from build123d import *

# Parameters (mm, degrees)
SKETCH1_R           = 12.5
BOSS_EXTRUDE1_DEPTH = 22.6
SKETCH2_R           = 13.5
BOSS_EXTRUDE2_DEPTH = 11.58
SKETCH9_W           = 1.365
SKETCH9_H           = 0.55
SKETCH4_R           = 2.575
MAGNETSLOT_DEPTH    = 1
NUTCUT_DEPTH        = 30.18
SKETCH7_R           = 3.5
NUTHOLE_DEPTH       = 15
SKETCH8_R           = 1.35
SCREWHOLE_DEPTH     = 40.150637287
CIRPATTERN1_COUNT   = 4
SKETCH11_W          = 15.473481632
SKETCH11_H          = 6.154945972
CUT_EXTRUDE1_DEPTH  = 34.488804099


with BuildPart() as part:
    # Sketch1 → Boss-Extrude1 (new body)
    with BuildSketch(Plane.XY):
        Circle(SKETCH1_R)
    extrude(amount=BOSS_EXTRUDE1_DEPTH)

    # Sketch2 → Boss-Extrude2 (add)
    with BuildSketch(Plane.XY):
        Circle(SKETCH2_R)
    extrude(amount=-BOSS_EXTRUDE2_DEPTH)

    # Sketch9 → Cut-Revolve1 (revolve, cut)
    with BuildSketch(Plane(origin=(0, 0, 0), x_dir=(0, 0, -1), z_dir=(1, 0, 0)), mode=Mode.PRIVATE) as cut_revolve1_sk:
        with Locations((-20.6825, -12.225)):
            Rectangle(SKETCH9_W, SKETCH9_H)
    revolve(cut_revolve1_sk.sketch.rotate(Axis((0, 0, 24.309), (0, 0, -1)), 270), axis=Axis((0, 0, 24.309), (0, 0, -1)), mode=Mode.SUBTRACT)

    # Sketch4 → MagnetSlot (cut)
    with BuildSketch(Plane.XY.offset(22.6)):
        Circle(SKETCH4_R)
    magnetslot = extrude(amount=-MAGNETSLOT_DEPTH, mode=Mode.SUBTRACT)

    # Sketch6 → NutCut (cut)
    with BuildSketch(Plane.XY.offset(22.6)):
        Polygon((6.206811366, 8.288877648), (3.362655934, 7.526788497), (2.600566782, 4.682633064), (4.682633064, 2.600566782), (7.526788497, 3.362655934), (8.288877648, 6.206811366), align=None)
    nutcut = extrude(amount=-NUTCUT_DEPTH, mode=Mode.SUBTRACT)

    # Sketch7 → NutHole (cut)
    with BuildSketch(Plane.XY.offset(22.6)):
        with Locations((5.444722215, 5.444722215)):
            Circle(SKETCH7_R)
    nuthole = extrude(amount=-NUTHOLE_DEPTH, mode=Mode.SUBTRACT)

    # Sketch8 → ScrewHole (cut, symmetric)
    with BuildSketch(Plane.XY.offset(22.6)):
        with Locations((5.444722215, 5.444722215)):
            Circle(SKETCH8_R)
    screwhole = extrude(amount=SCREWHOLE_DEPTH, both=True, mode=Mode.SUBTRACT)

    # CirPattern1: MagnetSlot, NutCut, NutHole, ScrewHole ×4 about axis
    cirpattern1_axis = Axis((0, 0, 0), (0, 0, 1))
    add([magnetslot.rotate(cirpattern1_axis, i * 360 / CIRPATTERN1_COUNT) for i in range(1, CIRPATTERN1_COUNT)], mode=Mode.SUBTRACT)
    add([nutcut.rotate(cirpattern1_axis, i * 360 / CIRPATTERN1_COUNT) for i in range(1, CIRPATTERN1_COUNT)], mode=Mode.SUBTRACT)
    add([nuthole.rotate(cirpattern1_axis, i * 360 / CIRPATTERN1_COUNT) for i in range(1, CIRPATTERN1_COUNT)], mode=Mode.SUBTRACT)
    add([screwhole.rotate(cirpattern1_axis, i * 360 / CIRPATTERN1_COUNT) for i in range(1, CIRPATTERN1_COUNT)], mode=Mode.SUBTRACT)

    # Sketch11 → Cut-Extrude1 (cut, through all)
    with BuildSketch(Plane(origin=(7.2, 0, 0), x_dir=(0, 0, -1), z_dir=(1, 0, 0))):
        with Locations((7.736740816, 0)):
            Rectangle(SKETCH11_W, SKETCH11_H)
    extrude(amount=CUT_EXTRUDE1_DEPTH, mode=Mode.SUBTRACT)


solid = part.part
Verification items for the finished model (mm, model axes). A direction names the side the tool comes from. Round coordinates to 2 decimals unless told otherwise and drop trailing zeros. Loops run counter-clockwise (first coordinate to the right, second up) from the corner with the lowest first, then second, coordinate; pieces in that order, holes last. Notation, with made-up numbers: (20, 65.25) - (33, 65.25) arc R27 ccw to (33, 92.25) - close; hole circle Ø6 at (-33, -6.75). An arc over 180 degrees is marked (long way). Use one line per item in the form item = value.
1. Section check C-C on x = 0. Record the cut outline in (y, z) (3 decimals).
A:
outline = (-13.5, -11.58) - (13.5, -11.58) - (13.5, 0) - (12.5, 0) - (12.5, 20) - (11.95, 20) - (11.95, 21.365) - (12.5, 21.365) - (12.5, 22.6) - (2.575, 22.6) - (2.575, 21.6) - (-2.575, 21.6) - (-2.575, 22.6) - (-12.5, 22.6) - (-12.5, 21.365) - (-11.95, 21.365) - (-11.95, 20) - (-12.5, 20) - (-12.5, 0) - (-13.5, 0) - close
2. Section check B-B on z = 1. Record the cut outline in (x, y), and give its area (3 significant figures).
A:
outline = circle Ø25 at (0, 0); hole (-8.29, -6.21) - (-6.21, -8.29) - (-3.36, -7.53) - (-2.6, -4.68) - (-4.68, -2.6) - (-7.53, -3.36) - close; hole (-8.29, 6.21) - (-7.53, 3.36) - (-4.68, 2.6) - (-2.6, 4.68) - (-3.36, 7.53) - (-6.21, 8.29) - close; hole (2.6, -4.68) - (3.36, -7.53) - (6.21, -8.29) - (8.29, -6.21) - (7.53, -3.36) - (4.68, -2.6) - close; hole (2.6, 4.68) - (4.68, 2.6) - (7.53, 3.36) - (8.29, 6.21) - (6.21, 8.29) - (3.36, 7.53) - close
area = 401 mm²
3. Access from +Z, -Z, +X, -X, +Y, -Y to the whole of each face (thin tool, end or side, straight path). Record for faces 1 (the flat face through (7.2, 0, -6)), 2 (the cylindrical face through (4.373, 4.623, -9.552)), 3 (the flat face through (-6, 7, -7.58)).
A:
face_1 = -Z, +X
face_2 = +Z, -Z
face_3 = +Z
4. Section check A-A on y = 0. Record the cut outline in (x, z) (3 decimals).
A:
outline = (-13.5, -11.58) - (7.2, -11.58) - (7.2, 0) - (12.5, 0) - (12.5, 20) - (11.95, 20) - (11.95, 21.365) - (12.5, 21.365) - (12.5, 22.6) - (2.575, 22.6) - (2.575, 21.6) - (-2.575, 21.6) - (-2.575, 22.6) - (-12.5, 22.6) - (-12.5, 21.365) - (-11.95, 21.365) - (-11.95, 20) - (-12.5, 20) - (-12.5, 0) - (-13.5, 0) - close
5. Draft check along Z on faces 4 (the flat face through (10, 3.077, -6)), 5 (the cylindrical face through (-1.556, -11.848, 20.673)), 6 (the flat face through (-7, -6, -7.58)). Enter one of: pulls with the +Z half, pulls with the -Z half, needs draft (parallel to the pull), parting line crosses it, or undercut.
A:
face_4 = needs draft
face_5 = undercut
face_6 = pulls with the +Z half
6. Gauge pin test, flat ends, axial feed: pin 1 Ø5.5 at (x, y) = (-5, -5) entering from +Z; pin 2 Ø1.6 at (x, y) = (9, -1) entering from -Z; pin 3 Ø6.5 at (x, z) = (10.5, -4.5) entering from +Y. Record the tip position at first contact, or that the pin passes through.
A:
pin_1 = 7.6
pin_2 = 0
pin_3 = 11.39
7. Scan lines: probe 1 along X at (y, z) = (4.75, -7.5); probe 2 along X at (y, z) = (5.5, -2); probe 3 along Y at (x, z) = (-7, 9.5). Record each from-to range of solid material in increasing order.
A:
probe_1 = -12.64 to -7.9, -2.62 to 2.62, 7.9 to 12.64
probe_2 = -12.33 to -8.1, -2.82 to 2.82, 8.1 to 12.33
probe_3 = -10.36 to -8.58, -2.31 to 2.31, 8.58 to 10.36
8. Section check D-D on z = 16.5. Record the cut outline in (x, y), and give its area (3 significant figures).
A:
outline = circle Ø25 at (0, 0); hole circle Ø7 at (-5.44, -5.44); hole circle Ø7 at (-5.44, 5.44); hole circle Ø7 at (5.44, -5.44); hole circle Ø7 at (5.44, 5.44)
area = 337 mm²
